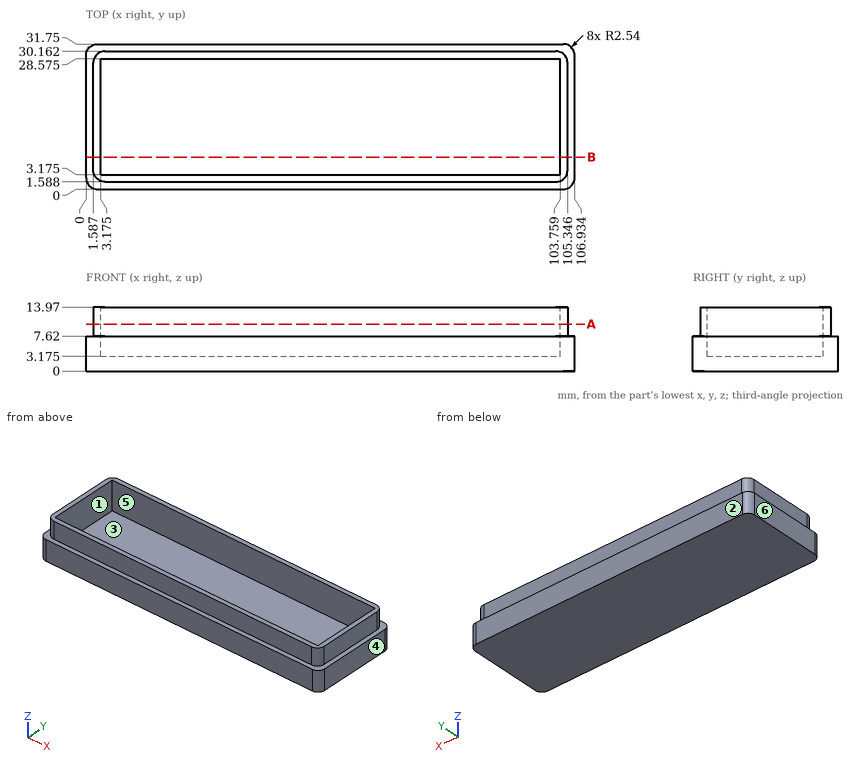
The figure shows three views and two pictorial views of one solid part (mm, origin at its lowest corner). Answer the questions. A direction names the side the tool comes from. Round coordinates to 2 decimals unless told otherwise and drop trailing zeros. Order: outer loops, then holes, each group sorted by start corner. A loop starts at its lowest first (then second) coordinate and runs counter-clockwise, first axis right, second up. Notation, with made-up numbers: (28.5, 83.5) -> (38.5, 83.5) arc R24 ccw to (38.5, 94.5) -> close; hole circle Ø7 at (35.5, 41.5). An arc over 180 degrees is marked (long way). Put each result on its own line as item: value.
Q1. Section B-B, the plane y = 7 is taken. Write down the section's boundary in (x, z) (1 decimal), and give its area (3 significant figures).
Results list:
outline: (0, 0) -> (106.9, 0) -> (106.9, 7.6) -> (105.3, 7.6) -> (105.3, 14) -> (103.8, 14) -> (103.8, 3.2) -> (3.2, 3.2) -> (3.2, 14) -> (1.6, 14) -> (1.6, 7.6) -> (0, 7.6) -> close
area: 388 mm^2
Q2. Which of the six approach directions +Z, -Z, +X, -X, +Y, -Y give full straight-line access (tool end or side, diameter ignored) to the marked faces 5 and 6?
Results list:
face 5: +Z
face 6: +Z, -Z, -X, +Y, -Y
Q3. Consider line 1 along X through (y, z) = (16, 6.5) (1 decimal); line 2 along X through (y, z) = (17.5, 8.75) (1 decimal); line 3 along Y through (x, z) = (10.5, 9.5) (1 decimal). Determine where each line is inside the solid, lowest interval first.
Results list:
line 1: 0 to 3.2, 103.8 to 106.9
line 2: 1.6 to 3.2, 103.8 to 105.3
line 3: 1.6 to 3.2, 28.6 to 30.2
Q4. Section A-A, the plane z = 10.25 is taken. Write down the section's boundary in (x, y) (1 decimal).
Results list:
outline: (1.6, 4.1) arc R2.5 ccw to (4.1, 1.6) -> (102.8, 1.6) arc R2.5 ccw to (105.3, 4.1) -> (105.3, 27.6) arc R2.5 ccw to (102.8, 30.2) -> (4.1, 30.2) arc R2.5 ccw to (1.6, 27.6) -> close; hole (3.2, 3.2) -> (103.8, 3.2) -> (103.8, 28.6) -> (3.2, 28.6) -> close
Q5. Determine the mould class of the marked faces 1, 2, 3 and 4 for opening direction X: pulls with the +X half, pulls with the -X half, needs draft (parallel to the pull), parting line crosses it, or undercut.
Results list:
face 1: undercut
face 2: needs draft
face 3: undercut
face 4: pulls with the +X half
Q6. Each of these flat-tipped pins is pushed along its axis until it touches: P1, Ø5, axis at y = 8.5, z = 3, coming from the -X side; P2, Ø16, axis at x = 50.5, y = 12, coming from the +Z side (1 decimal); P3, Ø3, axis at y = 11, z = 9.5, coming from the -X side; P4, Ø1, axis at x = 87.5, z = 10.5, coming from the +Y side. Where does it stop, or does it pass through?
Results list:
P1: x = 0
P2: z = 3.2
P3: x = 1.59
P4: y = 30.16
